Could you check a few things on this model? Use its own coordinates, in mm. A direction names the side the tool comes from. Round coordinates to 2 decimals unless told otherwise and drop trailing zeros. Loops run counter-clockwise (first coordinate to the right, second up) from the corner with the lowest first, then second, coordinate; pieces in that order, holes last. Notation, with made-up numbers: (36.25, 42) -> (56.25, 42) arc R18 cw to (56.25, 63) -> close; hole circle Ø10 at (-13, 87.25). An arc over 180 degrees is marked (long way). Write each question's results on one line, items separated by ' | '. Start each with the question number.
1) Imagine slicing it at A-A, the plane x = 16.5. List the corners of the cut face in (y, z) for me, plus the area to 3 significant figures.
2) If I drill on probe 1 along Y at (x, z) = (7.5, 46); probe 2 along X at (y, z) = (7.25, 11); probe 3 along Y at (x, z) = (29.5, 39.5), over which ranges is the centre line in solid material (lowest first)?
3) Imagine slicing it at B-B, the plane y = 7. List the corners of the cut face in (x, z) for me, plus the area to 3 significant figures.
4) Imagine slicing it at C-C, the plane z = 16.5. List the corners of the cut face in (x, y) for me.
5) We'd pull the mould along Y, two halves only. Please class faces 4 (the cylindrical face through (1, 12, 31)), 5 (the cylindrical face through (31, 13.9, 29.6)), 6 (the flat face through (33, 7, 30)), 7 (the flat face through (16.6, 1.8, 2)): pulls with the +Y half, pulls with the -Y half, needs draft (parallel to the pull), parting line crosses it, or undercut.
6) For P1, Ø1, axis at y = 15, z = 27, coming from the -X side; P2, Ø4, axis at y = 0, z = 47, coming from the +X side; P3, Ø1.6, axis at y = 15.5, z = 27, coming from the +X side, each with a flat end and sliding along its axis, tell me the tip position at first contact or that it passes through.
7) Imagine slicing it at D-D, the plane x = 9.5. List the corners of the cut face in (y, z) for me.
8) Which directions (+Z, -Z, +X, -X, +Y, -Y) give clear straight access to the entire face, cutting with the end or side of a thin tool? Please do faces 1 (the flat face through (15, 2, 1)), 2 (the cylindrical face through (30, 2, 31)), 3 (the flat face through (18.5, 15, 27)).
from build123d import *

# Parameters (mm, degrees)
F0_W     = 27
F0_H     = 10
F1_DEPTH = 2
F2_DEPTH = 60
F3_W     = 6
F3_H     = 3
F4_DEPTH = 25


with BuildPart() as f1:
    # F0 (on Top) → F1 (new body)
    with BuildSketch(Plane.XY):
        with BuildLine():
            Line((26, 16), (5, 16))
            ThreePointArc((5, 16), (0.0502525317, 13.9497474683), (-2, 9))
            Line((-2, 9), (-2, 5))
            ThreePointArc((-2, 5), (0.0502525317, 0.0502525317), (5, -2))
            Line((5, -2), (26, -2))
            ThreePointArc((26, -2), (30.9497474683, 0.0502525317), (33, 5))
            Line((33, 5), (33, 9))
            ThreePointArc((33, 9), (30.9497474683, 13.9497474683), (26, 16))
        make_face()
        with BuildLine():
            Line((26, 0), (5, 0))
            ThreePointArc((5, 0), (1.4644660941, 1.4644660941), (0, 5))
            Line((0, 5), (0, 9))
            ThreePointArc((0, 9), (1.4644660941, 12.5355339059), (5, 14))
            Line((5, 14), (26, 14))
            ThreePointArc((26, 14), (29.5355339059, 12.5355339059), (31, 9))
            Line((31, 9), (31, 5))
            ThreePointArc((31, 5), (29.5355339059, 1.4644660941), (26, 0))
        make_face(mode=Mode.SUBTRACT)
        with BuildLine():
            ThreePointArc((0, 5), (1.4644660941, 1.4644660941), (5, 0))
            Line((5, 0), (26, 0))
            ThreePointArc((26, 0), (29.5355339059, 1.4644660941), (31, 5))
            Line((31, 5), (31, 9))
            ThreePointArc((31, 9), (29.5355339059, 12.5355339059), (26, 14))
            Line((26, 14), (5, 14))
            ThreePointArc((5, 14), (1.4644660941, 12.5355339059), (0, 9))
            Line((0, 9), (0, 5))
        make_face()
        with Locations((15.5, 7)):
            Rectangle(F0_W, F0_H, mode=Mode.SUBTRACT)
    extrude(amount=F1_DEPTH)

    # F0 (on Top) → F2 (join)
    with BuildSketch(Plane.XY):
        with BuildLine():
            Line((26, 16), (5, 16))
            ThreePointArc((5, 16), (0.0502525317, 13.9497474683), (-2, 9))
            Line((-2, 9), (-2, 5))
            ThreePointArc((-2, 5), (0.0502525317, 0.0502525317), (5, -2))
            Line((5, -2), (26, -2))
            ThreePointArc((26, -2), (30.9497474683, 0.0502525317), (33, 5))
            Line((33, 5), (33, 9))
            ThreePointArc((33, 9), (30.9497474683, 13.9497474683), (26, 16))
        make_face()
        with BuildLine():
            Line((26, 0), (5, 0))
            ThreePointArc((5, 0), (1.4644660941, 1.4644660941), (0, 5))
            Line((0, 5), (0, 9))
            ThreePointArc((0, 9), (1.4644660941, 12.5355339059), (5, 14))
            Line((5, 14), (26, 14))
            ThreePointArc((26, 14), (29.5355339059, 12.5355339059), (31, 9))
            Line((31, 9), (31, 5))
            ThreePointArc((31, 5), (29.5355339059, 1.4644660941), (26, 0))
        make_face(mode=Mode.SUBTRACT)
    extrude(amount=F2_DEPTH)

    # F3 (on Front) → F4 (cut)
    with BuildSketch(Plane.XZ):
        with Locations((15.5, 26.5405690297)):
            Rectangle(F3_W, F3_H)
    extrude(amount=-F4_DEPTH, mode=Mode.SUBTRACT)


solid = f1.part
Checked values:
1) outline: (-2, 0) -> (2, 0) -> (2, 2) -> (0, 2) -> (0, 60) -> (-2, 60) -> close; (12, 0) -> (16, 0) -> (16, 25.04) -> (14, 25.04) -> (14, 2) -> (12, 2) -> close; (14, 28.04) -> (16, 28.04) -> (16, 60) -> (14, 60) -> close | area: 242 mm^2
2) probe 1: -2 to 0, 14 to 16 | probe 2: -2 to 0, 31 to 33 | probe 3: -1.06 to 1.43, 12.57 to 15.06
3) outline: (-2, 0) -> (2, 0) -> (2, 2) -> (0, 2) -> (0, 60) -> (-2, 60) -> close; (29, 0) -> (33, 0) -> (33, 60) -> (31, 60) -> (31, 2) -> (29, 2) -> close | area: 248 mm^2
4) outline: (-2, 5) arc R7 ccw to (5, -2) -> (26, -2) arc R7 ccw to (33, 5) -> (33, 9) arc R7 ccw to (26, 16) -> (5, 16) arc R7 ccw to (-2, 9) -> close; hole (0, 5) arc R5 ccw to (5, 0) -> (26, 0) arc R5 ccw to (31, 5) -> (31, 9) arc R5 ccw to (26, 14) -> (5, 14) arc R5 ccw to (0, 9) -> close
5) face 4: undercut | face 5: pulls with the +Y half | face 6: needs draft | face 7: undercut
6) P1: x = 0.67 | P2: x = 32.32 | P3: x = 30.06
7) outline: (-2, 0) -> (2, 0) -> (2, 2) -> (0, 2) -> (0, 60) -> (-2, 60) -> close; (12, 0) -> (16, 0) -> (16, 60) -> (14, 60) -> (14, 2) -> (12, 2) -> close
8) face 1: +Z, -Z | face 2: +Z | face 3: +Y
